Source: CAD feature listing. Evaluate the final solid. Frame: model axes, mm. A direction names the side the tool comes from. Round coordinates to 2 decimals unless told otherwise and drop trailing zeros. Loops run counter-clockwise (first coordinate to the right, second up) from the corner with the lowest first, then second, coordinate; pieces in that order, holes last. Notation, with made-up numbers: M 51,8 L 99,8 A34 ccw 99,39 Z; hole C 14.5,-1.75 d7. An arc over 180 degrees is marked long. Answer as a JSON object with one key per item and string values.
from build123d import *

# Parameters (mm, degrees)
F1_DEPTH = 10
F3_DEPTH = 6
F4_SIZE  = 1


with BuildPart() as f1:
    # F0 (on Top) → F1 (new body)
    with BuildSketch(Plane.XY):
        with BuildLine():
            Line((-15, 30), (-15, 0))
            Line((-15, 0), (-4.5, 0))
            Line((-4.5, 0), (-4.5, 15))
            ThreePointArc((-4.5, 15), (0, 19.5), (4.5, 15))
            Line((4.5, 15), (4.5, 0))
            Line((4.5, 0), (15, 0))
            Line((15, 0), (15, 30))
            Line((15, 30), (-15, 30))
        make_face()
    extrude(amount=F1_DEPTH)

    # F2 (on Top) → F3 (cut)
    with BuildSketch(Plane.XY):
        with BuildLine():
            Line((4.5, 0), (9.5, 0))
            Line((9.5, 0), (9.5, 15))
            ThreePointArc((9.5, 15), (0, 24.5), (-9.5, 15))
            Line((-9.5, 15), (-9.5, 0))
            Line((-9.5, 0), (-4.5, 0))
            Line((-4.5, 0), (-4.5, 15))
            ThreePointArc((-4.5, 15), (0, 19.5), (4.5, 15))
            Line((4.5, 15), (4.5, 0))
        make_face()
    extrude(amount=F3_DEPTH, mode=Mode.SUBTRACT)

    # F4
    f4_edges = [f1.edges().sort_by_distance(p)[0] for p in [
        (-9.5, 0, 3),
        (-4.5, 0, 8),
        (9.5, 0, 3),
        (4.5, 0, 8),
    ]]
    chamfer(f4_edges, length=F4_SIZE)


solid = f1.part
Item 1: Line query: probe 1 along X at (y, z) = (9.25, 1); probe 2 along X at (y, z) = (8, 7); probe 3 along Z at (x, y) = (7.75, 20.25). Output: solid intervals per line, ascending. Write a range as from..to.
Answer sheet:
{"probe 1": "x = -15..-9.5, 9.5..15", "probe 2": "x = -15..-4.5, 4.5..15", "probe 3": "z = 6..10"}
Item 2: Contact query for flat-ended pins moving along their axis: pin 1 Ø1 at (x, z) = (-7.5, 2.5) entering from -Y; pin 2 Ø6.5 at (x, y) = (3, 15.5) entering from -Z. Output: stop coordinate, or through.
Answer sheet:
{"pin 1": "stops at y = 20.12", "pin 2": "stops at z = 6"}
Item 3: Section A-A on y = 7. Return the cut outline in (x, z), then the cut area to 3 significant figures.
Answer sheet:
{"outline": "M -15,0 L -9.5,0 L -9.5,6 L -4.5,6 L -4.5,10 L -15,10 Z; M 4.5,6 L 9.5,6 L 9.5,0 L 15,0 L 15,10 L 4.5,10 Z", "area": "150 mm²"}
Item 4: Section C-C on z = 1. Return the cut outline in (x, y).
Answer sheet:
{"outline": "M -15,0 L -10.5,0 L -9.5,1 L -9.5,15 A9.5 cw 9.5,15 L 9.5,1 L 10.5,0 L 15,0 L 15,30 L -15,30 Z"}
Item 5: Section D-D on y = 18.5. Return the cut outline in (x, z), then the cut area to 3 significant figures.
Answer sheet:
{"outline": "M -15,0 L -8.83,0 L -8.83,6 L -2.83,6 L -2.83,10 L -15,10 Z; M 2.83,6 L 8.83,6 L 8.83,0 L 15,0 L 15,10 L 2.83,10 Z", "area": "171 mm²"}
Item 6: Section B-B on x = 0. Return the cut outline in (y, z).
Answer sheet:
{"outline": "M 19.5,6 L 24.5,6 L 24.5,0 L 30,0 L 30,10 L 19.5,10 Z"}
Item 7: Access query for faces 1 (the flat face through (4.5, 8, 8)), 2 (the flat face through (-9.5, 8, 3)), 3 (the flat face through (-11, 0, 6)). Directions: +Z, -Z, +X, -X, +Y, -Y. A direction counts if a zero-diameter tool reaches every point of the face in a straight line with its end or side. Return the directions, or none.
Answer sheet:
{"face 1": "+Z, -Z, -Y", "face 2": "-Z, -Y", "face 3": "+Z, -Z, +X, -X, -Y"}
Item 8: Pull-direction query (X, two-part tool) for faces 4 (the flat face through (-4, 19, 10)), 5 (the flat face through (15, 15, 5)), 6 (the flat face through (5, 0.5, 8)); classes: pulls with the +X half, pulls with the -X half, needs draft (parallel to the pull), parting line crosses it, or undercut.
Answer sheet:
{"face 4": "needs draft", "face 5": "pulls with the +X half", "face 6": "undercut"}
